Check sheet for the modelled part. Datum: model origin and axes. Units: mm. Face numbers are marked on the shaded views. A direction names the side the tool comes from. Round coordinates to 2 decimals unless told otherwise and drop trailing zeros. Order: outer loops, then holes, each group sorted by start corner. A loop starts at its lowest first (then second) coordinate and runs counter-clockwise, first axis right, second up.
Autodesk Inventor part; units mm, degrees
ref_plane "Arbeitsebene10" through (0, 0, 19) normal (0, 0, 1) x (1, 0, 0)
ref_plane "YZ Plane" through (0, 0, 0) normal (1, 0, 0) x (0, 1, 0)
ref_plane "XZ Plane" through (0, 0, 0) normal (0, 1, 0) x (-1, 0, 0)
sketch "Skizze1" plane through (0, 0, 0) normal (1, 0, 0) x (0, 1, 0)
  line L0 (0, 0) -> (0, 55)
  line L1 (44, 0) -> (0, 0) construction
  line L2 (3.1, 21) -> (3.1, 18)
  line L3 (44, 0) -> (40, 0)
  line L4 (40, 0) -> (40, -5)
  line L5 (40, -5) -> (44, -5)
  line L6 (44, -5) -> (44, 0)
  line L7 (3.1, 18) -> (40, 18)
  line L8 (40, 18) -> (40, 0)
  line L9 (3.1, 21) -> (44, 21)
  line L10 (44, 21) -> (44, 0)
  point P0 (21.7075, 15.1998)
  dimension "d143" = 6.2
  dimension "d146" = 18
  dimension "d147" = 3
  dimension "d155" = 5
  dimension "d156" = 4
  dimension "d186" = 80
revolve "Umdrehung4" add sketch "Skizze1" angle 360 about axis through (0, 0, 0) along (0, 0, 1)
sketch "Skizze28" plane through (0, 0, -5) normal (0, 0, -1) x (-1, 0, 0)
  circle A0 centre (0, 0) radius 44
  circle A1 centre (0, 0) radius 40
  circle A2 centre (0, 0) radius 51
  dimension "d157" = 102
extrude "Extrusion10" add sketch "Skizze28" against normal blind 7 contours A0 | A2
sketch "Skizze29" plane through (0, 0, -5) normal (0, 0, -1) x (-1, 0, 0)
  circle A0 centre (0, 0) radius 51
  circle A1 centre (0, 0) radius 43
  dimension "d160" = 86
extrude "Extrusion11" cut sketch "Skizze29" against normal blind 3.5
sketch "Skizze30" plane through (0, 0, -1.5) normal (0, 0, -1) x (-1, 0, 0)
  circle A0 centre (0, 0) radius 43
  circle A1 centre (0, 0) radius 51
  point P0 (-48, 0)
  dimension "d163" = 48
hole "Bohrung3" at (48, 0, -1.5) direction (0, 0, 1) diameter 3.3 end through all
pattern_circular "Runde Anordnung2" count 6 over 360 about axis through (0, 0, -5) along (0, 0, 1) of "Bohrung3"
ref_plane "Arbeitsebene10" through (0, 0, 19) normal (0, 0, 1) x (1, 0, 0)
fillet "Rundung1" radius 15 1 edges at (0, -40, 18)
fillet "Rundung2" radius 18 1 edges at (0, -44, 21)
properties part number "Kugel_oben_V5_Riza" material "ABS-Kunststoff"
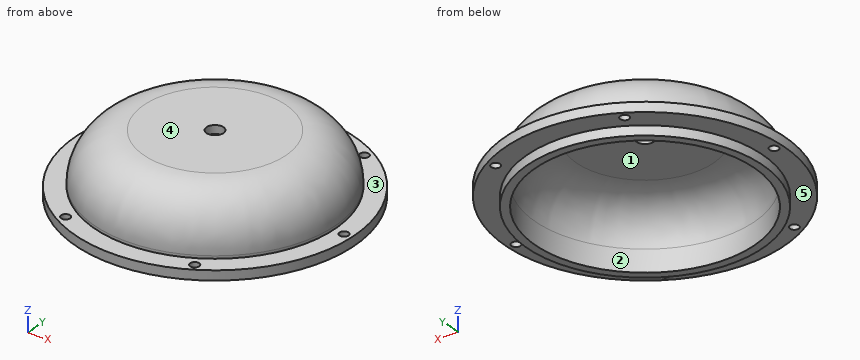
Item 1: Sectioned sample at A-A (x = 0). Record the cut outline in (y, z), and give its area (3 significant figures).
Answer:
outline: (-51, -1.5) - (-43, -1.5) - (-43, -5) - (-40, -5) - (-40, 3) arc R15 cw to (-25, 18) - (-3.1, 18) - (-3.1, 21) - (-26, 21) arc R18 ccw to (-44, 3) - (-44, 2) - (-51, 2) - close; (3.1, 18) - (25, 18) arc R15 cw to (40, 3) - (40, -5) - (43, -5) - (43, -1.5) - (51, -1.5) - (51, 2) - (44, 2) - (44, 3) arc R18 ccw to (26, 21) - (3.1, 21) - close
area: 429 mm2
Item 2: Release check for a two-part mould opening along X. For the marked faces 1, 2 and 3 record: released by +X, released by -X, zero draft, split by the parting line, or undercut.
Answer:
face 1: undercut
face 2: undercut
face 3: zero draft
Item 3: Access from +Z, -Z, +X, -X, +Y, -Y to the whole of each face (thin tool, end or side, straight path). Record for the marked faces 4 and 5.
Answer:
face 4: +Z, +X, -X, +Y, -Y
face 5: -Z
Item 4: Sectioned sample at D-D (z = 12.5). Record the cut outline in (x, y).
Answer:
outline: circle Ø82.58 at (0, 0); hole circle Ø73.22 at (0, 0)
Item 5: Scan lines: line 1 along Y through (x, z) = (0, 0.75); line 2 along Z through (x, y) = (32.5, 35.5); line 3 along Y through (x, z) = (-2, -2.25). Record each from-to range of solid material in increasing order.
Answer:
line 1: y = -51 to -40, 40 to 51
line 2: z = -1.5 to 2
line 3: y = -42.95 to -39.95, 39.95 to 42.95
Item 6: Go/stop test with flat-tipped pins: P1, Ø1, axis at y = 37.5, z = 11.5, coming from the -X side; P2, Ø8, axis at x = -5, y = 33, coming from the -Z side; P3, Ø2.5, axis at x = 24, y = -41.57, coming from the +Z side; P4, Ø4, axis at x = 31, y = -25, coming from the +Z side. Record where each tip stops, or that it passes through.
Answer:
P1: stops at x = -19.75
P2: stops at z = 11.47
P3: passes through
P4: stops at z = 16.57
Item 7: Sectioned sample at C-C (x = 48). Record the cut outline in (y, z).
Answer:
outline: (-17.23, -1.5) - (-1.65, -1.5) - (-1.65, 2) - (-17.23, 2) - close; (1.65, -1.5) - (17.23, -1.5) - (17.23, 2) - (1.65, 2) - close
Item 8: Sectioned sample at B-B (y = 0). State how many separate pieces and enclosed holes the cut face has, and give its area (3 significant figures).
Answer:
separate pieces: 4
enclosed holes: 0
area: 406 mm2
